Input: dimensioned drawing with shaded views. Units: mm. Origin: part minimum x, y, z. Coordinates: 2 decimals unless noted, no trailing zeros. Write each loop counter-clockwise with the first axis right and the second up, starting at its lowest first coordinate (ties: lowest second). Pieces come first, ordered by that corner, then holes. Notation, with made-up numbers: M 66.25,-19 L 122.25,-19 A14 cw 122.25,-3 Z; hole C -27,-11.5 d10. An arc over 180 degrees is marked long. Use one line per item in the form item = value.
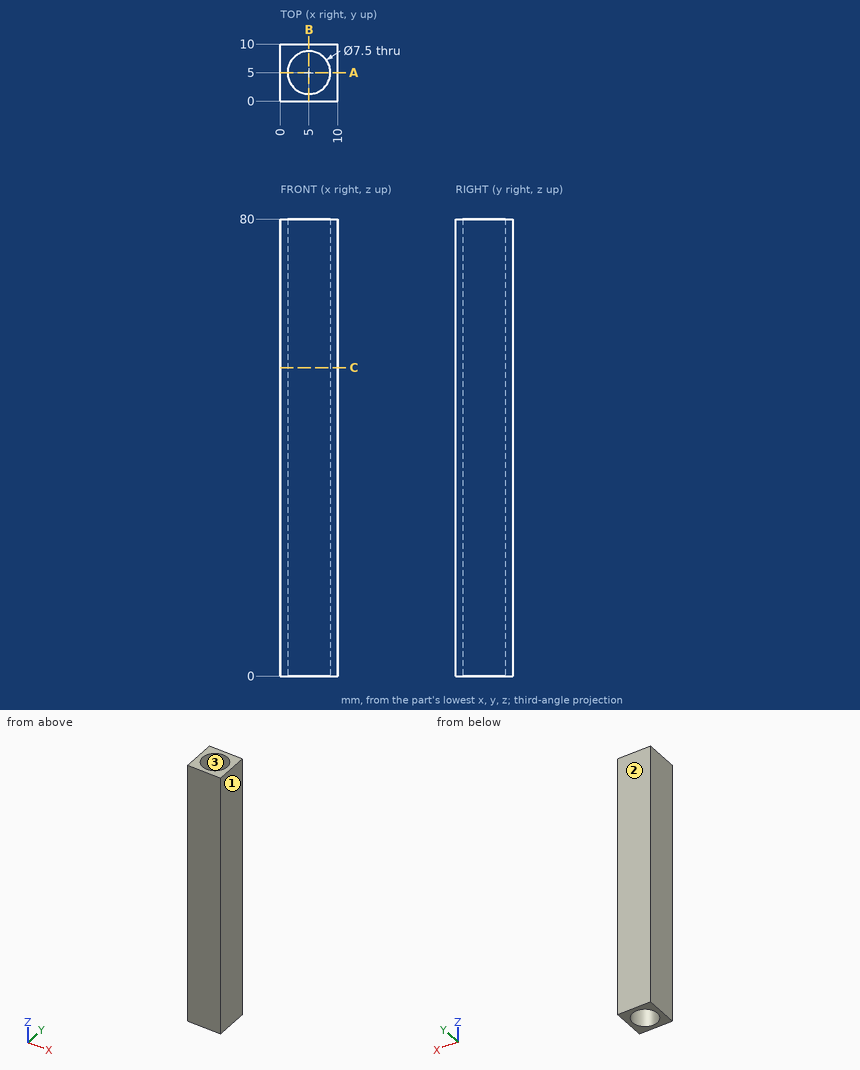
(1) Section query C-C on z = 54. Return the cut outline in (x, y), plus the area to 3 significant figures.
Computed:
outline = M 0,0 L 10,0 L 10,10 L 0,10 Z; hole C 5,5 d7.5
area = 55.8 mm^2
(2) First-contact query: pin 1 Ø4 at (y, z) = (4, 34.5) entering from -X. Flat tip, straight axial feed; report the tip coordinate or a pass-through.
Computed:
pin_1 = 0
(3) Section query A-A on y = 5. Return the cut outline in (x, z).
Computed:
outline = M 0,0 L 1.25,0 L 1.25,80 L 0,80 Z; M 8.75,0 L 10,0 L 10,80 L 8.75,80 Z
(4) Pull-direction query (X, two-part tool) for the marked faces 1, 2 and 3; classes: pulls with the +X half, pulls with the -X half, needs draft (parallel to the pull), parting line crosses it, or undercut.
Computed:
face_1 = pulls with the +X half
face_2 = needs draft
face_3 = undercut
(5) Line query: probe 1 along X at (y, z) = (5.25, 15); probe 2 along X at (y, z) = (7.5, 70). Output: solid intervals per line, ascending.
Computed:
probe_1 = 0 to 1.26, 8.74 to 10
probe_2 = 0 to 2.2, 7.8 to 10
